from build123d import *

# Parameters (mm, degrees)
F4_DEPTH = 360


with BuildPart() as f2:
    # F2: sweep along a path in F0
    with BuildLine(Plane.XZ) as f2_path:
        ThreePointArc((242.7527745604, 20.7435647383), (128.2776322592, 35.2070479661), (16.1666904568, 7.9144247848))
    # F1 (on Right) → F2 (sweep)
    with BuildSketch(Plane.YZ):
        Polygon((-320, 0), (0, 0), (320, 0), (0, 9.1953519732), align=None)
    sweep(path=f2_path.line)

    # F3: sweep along a path in F0
    with BuildLine(Plane.XZ) as f3_path:
        ThreePointArc((-242.7527745604, -20.7435647383), (-128.2776322592, -35.2070479661), (-16.1666904568, -7.9144247848))
    # F1 (on Right) → F3 (sweep)
    with BuildSketch(Plane.YZ):
        Polygon((320, 0), (0, 0), (-320, 0), (0, -9.1953519732), align=None)
    sweep(path=f3_path.line)

    # F0 (on Front) → F4 (join, symmetric)
    with BuildSketch(Plane.XZ):
        with BuildLine():
            ThreePointArc((-16.1666904568, -7.9144247848), (4.061992847, -17.5356840218), (18, 0))
            ThreePointArc((18, 0), (17.5356840218, 4.061992847), (16.1666904568, 7.9144247848))
            ThreePointArc((16.1666904568, 7.9144247848), (-7.9144247848, 16.1666904568), (-16.1666904568, -7.9144247848))
        make_face()
    extrude(amount=F4_DEPTH, both=True)


solid = f2.part
Check sheet for the modelled part. Datum: model origin and axes. Units: mm. Give positions to 0.01 mm unless a question says otherwise; leave off trailing zeros. Write each loop counter-clockwise with the first axis right and the second up, starting at its lowest first coordinate (ties: lowest second). Pieces come first, ordered by that corner, then holes. Notation, with made-up numbers: M 45,9.5 L 58,9.5 A3 ccw 58,14.5 Z; hole C -10,68 d9. An arc over 180 degrees is marked long. Use one line per item in the form item = value.
(1) Section check A-A on x = 0. Record the boundary of the cut face in (y, z).
Answer block:
outline = M -360,-18 L 360,-18 L 360,18 L -360,18 Z
(2) Draft check along X on faces 1 (the cylindrical face through (-120.8, -4.48, -34.59)), 2 (the flat face through (0, -360, 0)). Enter one of: pulls with the +X half, pulls with the -X half, needs draft (parallel to the pull), parting line crosses it, or undercut.
Answer block:
face_1 = undercut
face_2 = needs draft
(3) Depth check by flat-ended pin: P1, Ø10, axis at x = 39, y = -42, coming from the -Z side; P2, Ø12, axis at x = -147.5, y = -233, coming from the -Z side; P3, Ø2, axis at x = 79.5, y = -59, coming from the +Z side. Enter the tip coordinate at first touch or a pass-through.
Answer block:
P1 = 15.15
P2 = -37.98
P3 = 35.56
(4) Material ranges on line 1 along X through (y, z) = (194, -11); line 2 along X through (y, z) = (81, -3); line 3 along X through (y, z) = (261.5, 8), recorded low to high.
Answer block:
line_1 = -23.57 to -15.44, -14.25 to 14.25
line_2 = -17.75 to 17.75
line_3 = -16.12 to 16.62
